from build123d import *

# Parameters (mm, degrees)
F1_DEPTH = 11.5


with BuildPart() as f1:
    # F0 (on Top) → F1 (new body)
    with BuildSketch(Plane.XY):
        with BuildLine():
            ThreePointArc((4.609772, -3), (5.272748, -1.564649), (5.5, 0))
            ThreePointArc((5.5, 0), (5.272748, 1.564649), (4.609772, 3))
            ThreePointArc((4.609772, 3), (-5.5, 0), (4.609772, -3))
        make_face()
        with BuildLine():
            ThreePointArc((4.609772, 3), (5.272748, 1.564649), (5.5, 0))
            ThreePointArc((5.5, 0), (5.272748, -1.564649), (4.609772, -3))
            Line((4.609772, -3), (19.390228, -3))
            ThreePointArc((19.390228, -3), (18.5, 0), (19.390228, 3))
            Line((19.390228, 3), (4.609772, 3))
        make_face()
        with BuildLine():
            ThreePointArc((29.5, 0), (25.564649, 5.272748), (19.390228, 3))
            ThreePointArc((19.390228, 3), (18.5, 0), (19.390228, -3))
            ThreePointArc((19.390228, -3), (25.564649, -5.272748), (29.5, 0))
        make_face()
    extrude(amount=F1_DEPTH)


solid = f1.part
The model under review builds one solid part; all positions refer to its coordinate system, in mm. A direction names the side the tool comes from. Give positions to 0.01 mm unless a question says otherwise; leave off trailing zeros. Order: outer loops, then holes, each group sorted by start corner. A loop starts at its lowest first (then second) coordinate and runs counter-clockwise, first axis right, second up. Notation, with made-up numbers: M 25.25,57 L 31.25,57 A32 ccw 31.25,84 Z; hole C -18,43.25 d10. An arc over 180 degrees is marked long. Use one line per item in the form item = value. Start each with the question number.
Item 1: The part is to be moulded in two halves that separate along X. For faces 1 (the flat face through (12, 0, 11.5)), 2 (the flat face through (12, 3, 6)), 3 (the cylindrical face through (-5.496, 0.197, 5.67)), say which applies: pulls with the +X half, pulls with the -X half, needs draft (parallel to the pull), parting line crosses it, or undercut.
Item 2: For faces 4 (the flat face through (12, 0, 0)), 5 (the flat face through (12, -3, 6)), list the 3-axis set-ups (+Z, -Z, +X, -X, +Y, -Y) from which the entire face can be reached by the end or side of a thin tool; tool diameter is ignored.
Item 3: We need section B-B on z = 5. Give the boundary of the cut face in (x, y), plus the area to 3 significant figures.
Item 4: We need section C-C on x = 5.5. Give the boundary of the cut face in (y, z), plus the area to 3 significant figures.
Item 5: We need section D-D on y = -5. Give the boundary of the cut face in (x, z), plus the area to 3 significant figures.
Item 6: To check wall thickness, follow line 1 along Y through (x, z) = (14, 6.5); line 2 along X through (y, z) = (-0.25, 1.5); line 3 along X through (y, z) = (4.75, 4). State the ranges of each line that lie inside material, in increasing order. Write a range as from..to.
Item 7: We need section A-A on y = 3.75. Give the boundary of the cut face in (x, z), plus the area to 3 significant figures.
Item 8: Insertion check: pin 1 Ø2 at (x, z) = (11.5, 6) entering from -Y; pin 2 Ø1 at (y, z) = (2, 2) entering from +X; pin 3 Ø3 at (x, z) = (18, 7) entering from +Y. Each pin has a flat end and moves straight along its axis. Give the tip position at first contact, or say it passes through.
Completed:
q1.face_1 = needs draft
q1.face_2 = undercut
q1.face_3 = undercut
q2.face_4 = -Z, +X, -X, +Y, -Y
q2.face_5 = +Z, -Z, -Y
q3.outline = M 4.61,-3 L 19.39,-3 A5.5 ccw long 19.39,3 L 4.61,3 A5.5 ccw long Z
q3.area = 272 mm²
q4.outline = M -3,0 L 3,0 L 3,11.5 L -3,11.5 Z
q4.area = 69.0 mm²
q5.outline = M -2.29,0 L 2.29,0 L 2.29,11.5 L -2.29,11.5 Z; M 21.71,0 L 26.29,0 L 26.29,11.5 L 21.71,11.5 Z
q5.area = 105 mm²
q6.line_1 = -3..3
q6.line_2 = -5.49..29.49
q6.line_3 = -2.77..2.77, 21.23..26.77
q7.outline = M -4.02,0 L 4.02,0 L 4.02,11.5 L -4.02,11.5 Z; M 19.98,0 L 28.02,0 L 28.02,11.5 L 19.98,11.5 Z
q7.area = 185 mm²
q8.pin_1 = -3
q8.pin_2 = 29.29
q8.pin_3 = 3.16
